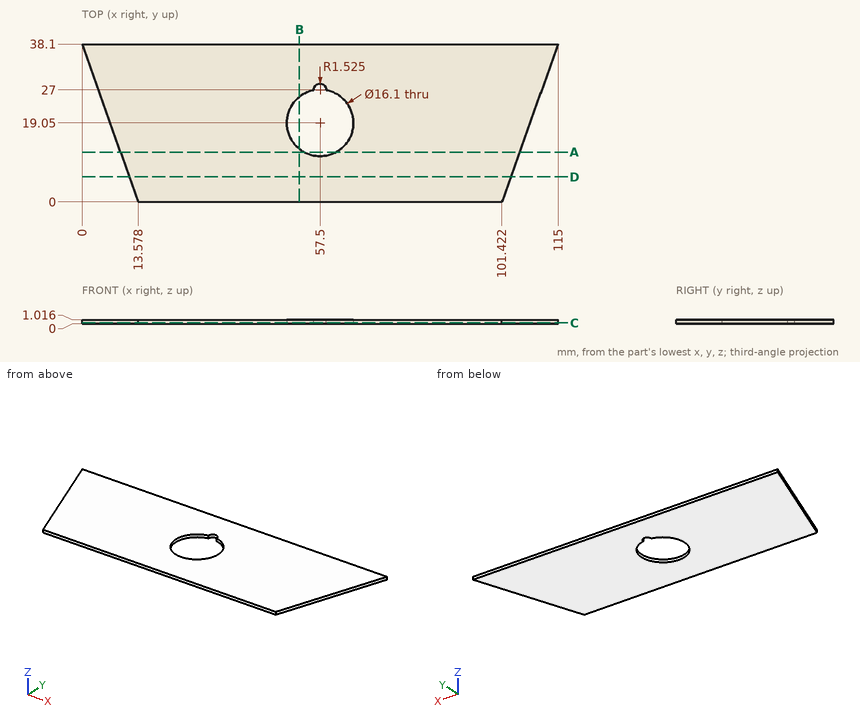
Source: three-view drawing plus pictorial views. Frame: mm from the lowest corner of the part. Round coordinates to 2 decimals unless told otherwise and drop trailing zeros. Loops run counter-clockwise (first coordinate to the right, second up) from the corner with the lowest first, then second, coordinate; pieces in that order, holes last.
Q1. Pin query (flat end, axial travel): P1, Ø4, axis at x = 56, y = 13.5, coming from the +Z side. Return the tip coordinate at first contact, or that it passes through.
Q2. Section D-D on y = 6. Return loops of the section in (x, z), plus the area to 3 significant figures.
Q3. Section A-A on y = 12. Return loops of the section in (x, z).
Q4. Section C-C on z = 0.25. Return loops of the section in (x, y) (3 decimals), plus the area to 3 significant figures.
Q5. Section B-B on x = 52.5. Return loops of the section in (y, z).
Q6. Material intervals for L1, parallel to Y at x = 57.5, z = 0.5 (3 decimals); L2, parallel to X at y = 16, z = 0.2; L3, parallel to X at y = 22.5, z = 0.2, sorted ascending.
Evaluation:
1. P1: passes through
2. outline: (11.44, 0) - (103.56, 0) - (103.56, 1.02) - (11.44, 1.02) - close
2. area: 93.6 mm2
3. outline: (9.3, 0) - (53.61, 0) - (53.61, 1.02) - (9.3, 1.02) - close; (61.39, 0) - (105.7, 0) - (105.7, 1.02) - (61.39, 1.02) - close
4. outline: (0, 38.1) - (13.578, 0) - (101.422, 0) - (115, 38.1) - close; hole (55.976, 26.954) arc R8.05 ccw (long way) to (59.024, 26.954) arc R1.525 ccw (long way) to start
4. area: 3,660 mm2
5. outline: (0, 0) - (12.74, 0) - (12.74, 1.02) - (0, 1.02) - close; (25.36, 0) - (38.1, 0) - (38.1, 1.02) - (25.36, 1.02) - close
6. L1: y = 0 to 11, 28.525 to 38.1
6. L2: x = 7.88 to 50.05, 64.95 to 107.12
6. L3: x = 5.56 to 50.23, 64.77 to 109.44
